Input: part model. Units: mm. Frame: model coordinates. A direction names the side the tool comes from. Give positions to 0.01 mm unless a question says otherwise; leave off trailing zeros. Order: outer loops, then holes, each group sorted by start corner. A loop starts at its lowest first (then second) coordinate and runs counter-clockwise, first axis right, second up. Notation, with made-up numbers: (-37.5, -24) -> (8.5, -24) arc R23 cw to (8.5, 12) -> close; hole circle Ø2 at (-8, -36.5). An arc over 180 degrees is marked (long way). Use a Markdown table: item, result. Add a question column.
from build123d import *

# Parameters (mm, degrees)
SKETCH1_W           = 120
SKETCH1_H           = 30
BOSS_EXTRUDE1_DEPTH = 3.175
SKETCH2_R           = 2
SKETCH2_R_2         = 4.5
CUT_EXTRUDE1_DEPTH  = 3.175
SKETCH3_W           = 22.072613883
SKETCH3_H           = 3.175
BOSS_EXTRUDE2_DEPTH = 63
SKETCH4_R           = 1.381817411
CUT_EXTRUDE2_DEPTH  = 10
SKETCH5_W           = 20.875808172
SKETCH5_H           = 3.175
BOSS_EXTRUDE3_DEPTH = 50


with BuildPart() as part:
    # Sketch1 → Boss-Extrude1 (new body)
    with BuildSketch(Plane(origin=(0, 0, 0), x_dir=(1, 0, 0), z_dir=(0, 1, 0))):
        with Locations((60, 15)):
            Rectangle(SKETCH1_W, SKETCH1_H)
    extrude(amount=BOSS_EXTRUDE1_DEPTH)

    # Sketch2 → Cut-Extrude1 (cut)
    with BuildSketch(Plane(origin=(0, 3.175, 0), x_dir=(1, 0, 0), z_dir=(0, 1, 0))):
        with Locations(Location((18, 15, 0), (0, 0, 270))):
            Circle(SKETCH2_R)
        with Locations(Location((100, 15, 0), (0, 0, 270))):
            Circle(SKETCH2_R_2)
    extrude(amount=-CUT_EXTRUDE1_DEPTH, mode=Mode.SUBTRACT)

    # Sketch3 → Boss-Extrude2 (add)
    with BuildSketch(Plane(origin=(0, 0, -30), x_dir=(-1, 0, 0), z_dir=(0, 0, -1))):
        with Locations((-108.963693059, 1.5875)):
            Rectangle(SKETCH3_W, SKETCH3_H)
    extrude(amount=BOSS_EXTRUDE2_DEPTH)

    # Sketch4 → Cut-Extrude2 (cut)
    with BuildSketch(Plane(origin=(0, 3.175, 0), x_dir=(1, 0, 0), z_dir=(0, 1, 0))):
        with Locations(Location((101.927386117, 71, 0), (0, 0, 270))):
            Circle(SKETCH4_R)
    extrude(amount=-CUT_EXTRUDE2_DEPTH, mode=Mode.SUBTRACT)

    # Sketch5 → Boss-Extrude3 (add)
    with BuildSketch(Plane.ZY.offset(-97.927386117)):
        with Locations((-82.562095914, 1.5875)):
            Rectangle(SKETCH5_W, SKETCH5_H)
    extrude(amount=BOSS_EXTRUDE3_DEPTH)


solid = part.part
Q1. Section query A-A (x = 18). Return loops of the section in (y, z) (3 decimals).
Q2. First-contact query: pin 1 (1.6 mm diameter, centred on x = 65.5, y = 2, fed in from +Z); pin 2 (1.6 mm diameter, centred on y = 1, z = -87.5, fed in from -X); pin 3 (1 mm diameter, centred on y = 2.5, z = -59, fed in from -X). Flat tips, straight axial feed; report the tip coordinate or a pass-through.
Q3. Access query for faces 5 (the flat face through (73, 2, -72.124)), 6 (the flat face through (47.927, 2, -83)), 7 (the flat face through (120, 2, -46)). Directions: +Z, -Z, +X, -X, +Y, -Y. A direction counts if a zero-diameter tool reaches every point of the face in a straight line with its end or side. Return the directions, or none.
Q4. Section query B-B (z = -15). Return loops of the section in (x, y) (3 decimals).
Q5. Section query D-D (x = 78). Return loops of the section in (y, z) (3 decimals).
Q6. Ray query, line 1 (X direction, y = 1.1, z = -15); line 2 (Z direction, x = 71, y = 2.5); line 3 (Z direction, x = 45.5, y = 1.4). Return the intervals inside material, ascending.
Q7. Draft query along X for faces 1 (the flat face through (0, 2, -15)), 2 (the cylindrical face through (20, 2, -15)), 3 (the cylindrical face through (103.093, 1.61, -70.257)), 4 (the flat face through (74, 3.175, -26)). Return one class per face: +X half, -X half, draft (parallel to the pull), parting line (faces both ways), or undercut.
Q8. Section query C-C (y = 1.65). Return loops of the section in (x, z).
Solution:
| question | item | result |
|---|---|---|
| 1 | outline | (0, -30) -> (3.175, -30) -> (3.175, -17) -> (0, -17) -> close; (0, -13) -> (3.175, -13) -> (3.175, 0) -> (0, 0) -> close |
| 2 | pin 1 | stops at z = 0 |
| 2 | pin 2 | stops at x = 47.93 |
| 2 | pin 3 | stops at x = 97.93 |
| 3 | face 5 | -X, +Y, -Y |
| 3 | face 6 | -Z, -X, +Y, -Y |
| 3 | face 7 | +Z, -Z, +X, +Y, -Y |
| 4 | outline | (0, 0) -> (16, 0) -> (16, 3.175) -> (0, 3.175) -> close; (20, 0) -> (95.5, 0) -> (95.5, 3.175) -> (20, 3.175) -> close; (104.5, 0) -> (120, 0) -> (120, 3.175) -> (104.5, 3.175) -> close |
| 5 | outline | (0, -93) -> (3.175, -93) -> (3.175, -72.124) -> (0, -72.124) -> close; (0, -30) -> (3.175, -30) -> (3.175, 0) -> (0, 0) -> close |
| 6 | line 1 | x = 0 to 16, 20 to 95.5, 104.5 to 120 |
| 6 | line 2 | z = -93 to -72.12, -30 to 0 |
| 6 | line 3 | z = -30 to 0 |
| 7 | face 1 | -X half |
| 7 | face 2 | undercut |
| 7 | face 3 | undercut |
| 7 | face 4 | draft |
| 8 | outline | (0, -30) -> (97.93, -30) -> (97.93, -72.12) -> (47.93, -72.12) -> (47.93, -93) -> (120, -93) -> (120, 0) -> (0, 0) -> close; hole circle Ø4 at (18, -15); hole circle Ø9 at (100, -15); hole circle Ø2.76 at (101.93, -71) |
